The model under review builds one solid part; all positions refer to its coordinate system, in mm. Give positions to 0.01 mm unless a question says otherwise; leave off trailing zeros. Order: outer loops, then holes, each group sorted by start corner. A loop starts at its lowest first (then second) coordinate and runs counter-clockwise, first axis right, second up.
```python
from build123d import *

# Parameters (mm, degrees)
SKETCH_1_R      = 2.6
EXTRUDE_1_DEPTH = 3.9
FILLET_1_R      = 0.5


with BuildPart() as part:
    # 草图1 → 凸台-拉伸1 (new body)
    with BuildSketch(Plane.XY):
        Polygon((4.618802154, 0), (2.309401077, 4), (-2.309401077, 4), (-4.618802154, 0), (-2.309401077, -4), (2.309401077, -4), align=None)
        Circle(SKETCH_1_R, mode=Mode.SUBTRACT)
    extrude(amount=EXTRUDE_1_DEPTH)

    # 圆角1
    fillet_1_edges = [part.edges().sort_by_distance(p)[0] for p in [
        (0, 4, 3.9),
        (-3.464101615, 2, 3.9),
        (-2.6, 0, 0),
        (-2.6, 0, 3.9),
        (-3.464101615, -2, 3.9),
        (0, -4, 3.9),
        (3.464101615, -2, 3.9),
        (0, -4, 0),
        (-3.464101615, -2, 0),
        (-3.464101615, 2, 0),
        (0, 4, 0),
        (3.464101615, 2, 0),
        (3.464101615, -2, 0),
        (3.464101615, 2, 3.9),
    ]]
    fillet(fillet_1_edges, radius=FILLET_1_R)


solid = part.part
```
Item 1: Draft analysis for pull direction X (two halves, no side actions). For faces 1 (the cylindrical face through (-3.36, 1.9, 3.75)), 2 (the cylindrical face through (-0.338, 2.578, 1.93)), 3 (the flat face through (3.448, -2.028, 1.93)), state which applies: released by +X, released by -X, zero draft, split by the parting line, or undercut.
Values found:
face 1: released by -X
face 2: undercut
face 3: released by +X
Item 2: Take a section at A-A (x = 0). Give the boundary of the cut face in (y, z).
Values found:
outline: (-4, 0.5) arc R0.5 ccw to (-3.5, 0) - (-3.1, 0) arc R0.5 ccw to (-2.6, 0.5) - (-2.6, 3.4) arc R0.5 ccw to (-3.1, 3.9) - (-3.5, 3.9) arc R0.5 ccw to (-4, 3.4) - close; (2.6, 0.5) arc R0.5 ccw to (3.1, 0) - (3.5, 0) arc R0.5 ccw to (4, 0.5) - (4, 3.4) arc R0.5 ccw to (3.5, 3.9) - (3.1, 3.9) arc R0.5 ccw to (2.6, 3.4) - close
Item 3: For line 1 (Y direction, x = 0, z = 2.8); line 2 (X direction, y = 1.5, z = 1.3); line 3 (Y direction, x = -1.5, z = 2.1), list the stretches that pass through material, from the lowest coordinate up.
Values found:
line 1: y = -4 to -2.6, 2.6 to 4
line 2: x = -3.75 to -2.12, 2.12 to 3.75
line 3: y = -4 to -2.12, 2.12 to 4
Item 4: Take a section at B-B (z = 2.8). Give the boundary of the cut face in (x, y), and give its area (3 significant figures).
Values found:
outline: (-4.62, 0) - (-2.31, -4) - (2.31, -4) - (4.62, 0) - (2.31, 4) - (-2.31, 4) - close; hole circle Ø5.2 at (0, 0)
area: 34.2 mm2
Item 5: Clearance check with flat-ended pins moving along their axes: pin 1 Ø1.5 at (x, y) = (-0.5, -2.5) entering from -Z; pin 2 Ø1.5 at (y, z) = (-1, 0.5) entering from -X; pin 3 Ø2 at (x, z) = (3.5, 2.5) entering from +Y. State where each tip first meets the part, or that it passes through.
Values found:
pin 1: stops at z = 0
pin 2: stops at x = -4.47
pin 3: stops at y = 3.67
